Check sheet for the modelled part. Datum: model origin and axes. Units: mm. A direction names the side the tool comes from. Give positions to 0.01 mm unless a question says otherwise; leave off trailing zeros. Loops run counter-clockwise (first coordinate to the right, second up) from the corner with the lowest first, then second, coordinate; pieces in that order, holes last. Notation, with made-up numbers: (75.25, -12.75) - (86.25, -12.75) arc R18 ccw to (86.25, 20.25) - close; hole circle Ø10 at (80, -28). An arc over 180 degrees is marked (long way). Use one line per item in the form item = value.
from build123d import *

# Parameters (mm, degrees)
SKETCH_1_R             = 25
EXTRUDE_1_DEPTH        = 5
HOLE_WIZARD_M4_2_D     = 3.3
HOLE_WIZARD_M4_2_DEPTH = 10.1
HOLE_WIZARD_M4_2_TIP   = 0.991420021
HOLE_WIZARD_M4_4_D     = 3.3
HOLE_WIZARD_M4_4_DEPTH = 10.1
HOLE_WIZARD_M4_4_TIP   = 0.991420021


with BuildPart() as part:
    # 草图1 → 凸台-拉伸1 (new body)
    with BuildSketch(Plane(origin=(0, 0, 0), x_dir=(1, 0, 0), z_dir=(0, 1, 0))):
        Polygon((0, 78.229669783), (-68.248539171, -38.236345737), (68.248539171, -38.236345737), align=None)
        Polygon((0, 60), (16.409255523, 30.960045876), (-16.683374686, 30.960045876), align=None, mode=Mode.SUBTRACT)
        Polygon((34.572863234, -1.184638197), (50.982118757, -30.224592321), (17.889488548, -30.224592321), align=None, mode=Mode.SUBTRACT)
        Polygon((-18.741152763, -30.224592321), (-51.833782972, -30.224592321), (-35.150408286, -1.184638197), align=None, mode=Mode.SUBTRACT)
        Circle(SKETCH_1_R, mode=Mode.SUBTRACT)
    extrude(amount=EXTRUDE_1_DEPTH)

    # M4 螺纹孔2
    with Locations(Plane(origin=(0, 5, 0), x_dir=(1, 0, 0), z_dir=(0, 1, 0))):
        with Locations((-24.082253567, 14.284434295), (0, 28), (24.082253567, 14.284434295), (24.585652853, -13.39946543), (0, -28), (-24.585652853, -13.39946543)):
            Hole(HOLE_WIZARD_M4_2_D / 2, depth=HOLE_WIZARD_M4_2_DEPTH)
            with Locations((0, 0, -(HOLE_WIZARD_M4_2_DEPTH + HOLE_WIZARD_M4_2_TIP / 2))):  # 118° drill point
                Cone(0, HOLE_WIZARD_M4_2_D / 2, HOLE_WIZARD_M4_2_TIP, mode=Mode.SUBTRACT)

    # M4 螺纹孔4
    with Locations(Plane(origin=(0, 5, 0), x_dir=(1, 0, 0), z_dir=(0, 1, 0))):
        with Locations((59.458609482, -33.236345737), (0, 68.229669783), (-59.458609482, -33.236345737)):
            Hole(HOLE_WIZARD_M4_4_D / 2, depth=HOLE_WIZARD_M4_4_DEPTH)
            with Locations((0, 0, -(HOLE_WIZARD_M4_4_DEPTH + HOLE_WIZARD_M4_4_TIP / 2))):  # 118° drill point
                Cone(0, HOLE_WIZARD_M4_4_D / 2, HOLE_WIZARD_M4_4_TIP, mode=Mode.SUBTRACT)


solid = part.part
Item 1: Section check A-A on z = -3. Record the boundary of the cut face in (x, y).
Answer block:
outline = (-44.08, 0) - (-24.82, 0) - (-24.82, 5) - (-44.08, 5) - close; (24.82, 0) - (44.08, 0) - (44.08, 5) - (24.82, 5) - close
Item 2: Gauge pin test, flat ends, axial feed: P1, Ø2, axis at y = 3, z = 19, coming from the +X side; P2, Ø2.5, axis at x = 24.08, z = -14.28, coming from the -Y side; P3, Ø1, axis at y = 2.5, z = -29, coming from the +X side; P4, Ø1, axis at y = 3.5, z = -63.5, coming from the +X side. Record the tip position at first contact, or that the pin passes through.
Answer block:
P1 = 57.56
P2 = through
P3 = 29.14
P4 = 8.92
Item 3: Section check D-D on z = 28. Record the boundary of the cut face in (x, y), then the cut area to 3 significant figures.
Answer block:
outline = (-62.25, 0) - (-50.56, 0) - (-50.56, 5) - (-62.25, 5) - close; (-20, 0) - (-1.65, 0) - (-1.65, 5) - (-20, 5) - close; (1.65, 0) - (19.17, 0) - (19.17, 5) - (1.65, 5) - close; (49.73, 0) - (62.25, 0) - (62.25, 5) - (49.73, 5) - close
area = 300 mm2
Item 4: Access from +Z, -Z, +X, -X, +Y, -Y to the whole of each face (thin tool, end or side, straight path). Record for faces 1 (the face through (-27.06, 2.46, 15.5)), 2 (the face through (34.602, 2.465, -19.181)).
Answer block:
face_1 = +Y, -Y
face_2 = -Z, +X, +Y, -Y
Item 5: Section check B-B on x = 30. Record the boundary of the cut face in (y, z), then the cut area to 3 significant figures.
Answer block:
outline = (0, -27.03) - (5, -27.03) - (5, 9.14) - (0, 9.14) - close; (0, 30.22) - (5, 30.22) - (5, 38.24) - (0, 38.24) - close
area = 221 mm2
Item 6: Section check C-C on y = 4.25. Give the number of separate pieces and of enclosed holes in the cut face, then the cut area to 3 significant figures.
Answer block:
separate_pieces = 1
enclosed_holes = 13
area = 4,470 mm2
Item 7: Thickness scan on L1, parallel to X at y = 3.6, z = 19; L2, parallel to X at y = 4.7, z = -18; L3, parallel to Z at x = -48, y = 1.3. Record the ranges inside material, lowest first.
Answer block:
L1 = -56.98 to -45.39, -25.08 to -16.25, 16.25 to 24.34, 44.64 to 56.98
L2 = -35.29 to -17.35, 17.35 to 35.29
L3 = 3.68 to 23.55, 30.22 to 38.24
Item 8: Mould release check, pull along Z, two halves, no side actions. Record for faces 3 (the face through (0.215, 2.465, 26.364)), 4 (the face through (-5, 5, -25)), 5 (the face through (-33.647, 2.465, -20.812)): released by +Z, released by -Z, zero draft, split by the parting line, or undercut.
Answer block:
face_3 = undercut
face_4 = zero draft
face_5 = released by -Z
